Input: part model. Units: mm. Frame: model coordinates. A direction names the side the tool comes from. Coordinates: 2 decimals unless noted, no trailing zeros. Loops run counter-clockwise (first coordinate to the right, second up) from the corner with the lowest first, then second, coordinate; pieces in that order, holes last. Notation, with made-up numbers: (7, -17.75) - (32, -17.75) arc R6 cw to (32, -11.75) - close; hole circle Ø10 at (-27, -39.5). An arc over 180 degrees is marked (long way). Answer as CSV lines item,"result". Start each with the question number.
Autodesk Inventor part; units mm, degrees
ref_plane "YZ Plane" through (0, 0, 0) normal (1, 0, 0) x (0, 1, 0)
ref_plane "XZ Plane" through (0, 0, 0) normal (0, 1, 0) x (-1, 0, 0)
ref_plane "XY Plane" through (0, 0, 0) normal (0, 0, 1) x (1, 0, 0)
sketch "Sketch1" plane through (0, 0, 0) normal (0, 0, 1) x (1, 0, 0)
  circle A0 centre (0, 0) radius 40.5
  arc A1 (-25.4, 37.7504) -> (25.4, 37.7504) centre (0, 0) ccw
  line L0 (-25.4, 37.7504) -> (-25.4, 57.7504)
  line L1 (-25.4, 57.7504) -> (25.4, 57.7504)
  line L2 (25.4, 57.7504) -> (25.4, 37.7504)
  dimension "d1" = 5
  dimension "d9" = 20
extrude "Extrusion1" add sketch "Sketch1" along normal blind 12
sketch "Sketch2" plane through (-25.4, 57.7504, 0) normal (0, 1, 0) x (1, 0, 0)
  line L0 (0, -12) -> (50.8, -12)
  line L1 (50.8, -12) -> (50.8, 0)
  line L2 (50.8, 0) -> (0, 0)
  line L3 (0, 0) -> (0, -12)
  point P0 (25.4, 0)
extrude "Extrusion2" add sketch "Sketch2" along normal blind 12
sketch "Sketch3" plane through (0, 0, 12) normal (0, 0, 1) x (1, 0, 0)
  line L0 (-25.4, 37.7504) -> (-25.4, 69.7504)
  line L1 (25.4, 37.7504) -> (25.4, 69.7504)
  line L2 (-25.4, 69.7504) -> (25.4, 69.7504)
  line L3 (25.4, 69.7504) -> (25.4, 56.7504)
  line L4 (25.4, 56.7504) -> (-25.4, 56.7504)
  line L5 (-25.4, 56.7504) -> (-25.4, 69.7504)
  point P0 (0, 0)
  dimension "d12" = 13
extrude "Extrusion3" add sketch "Sketch3" along normal blind 17.2
sketch "Sketch4" plane through (0, 0, 29.2) normal (0, 0, 1) x (1, 0, 0)
  line L0 (25.4, 69.7504) -> (-25.4, 69.7504)
  line L1 (-25.4, 69.7504) -> (-25.4, 37.7504)
  circle A0 centre (0, 0) radius 8.5
  arc A1 (-25.4, 37.7504) -> (25.4, 37.7504) centre (0, 0) ccw
  arc A2 (-25.4, 37.7504) -> (25.4, 37.7504) centre (0, 0) ccw
  line L2 (25.4, 37.7504) -> (25.4, 69.7504)
  line L3 (25.4, 37.7504) -> (25.4, 69.7504)
  line L4 (25.4, 69.7504) -> (-25.4, 69.7504)
  dimension "d15" = 17
extrude "Extrusion4" add sketch "Sketch4" along normal blind 5
sketch "Sketch5" plane through (0, 0, 34.2) normal (0, 0, 1) x (1, 0, 0)
  arc A0 (-25.4, 37.7504) -> (25.4, 37.7504) centre (0, 0) ccw
  circle A1 centre (0, 0) radius 4.5
  line L0 (-25.4, 37.7504) -> (-25.4, 69.7504)
  line L1 (-25.4, 37.7504) -> (-25.4, 69.7504)
  line L2 (25.4, 69.7504) -> (-25.4, 69.7504)
  line L3 (-25.4, 69.7504) -> (25.4, 69.7504)
  line L4 (25.4, 69.7504) -> (25.4, 37.7504)
  dimension "d18" = 9
extrude "Extrusion5" add sketch "Sketch5" along normal blind 27
sketch "Sketch6" plane through (0, 0, 61.2) normal (0, 0, 1) x (1, 0, 0)
  line L0 (25.4, 69.7504) -> (-25.4, 69.7504)
  line L1 (-25.4, 56.7504) -> (-25.4, 37.7504)
  line L2 (-25.4, 69.7504) -> (-25.4, 37.7504)
  line L3 (-25.4, 69.7504) -> (25.4, 69.7504)
  arc A0 (-25.4, 37.7504) -> (25.4, 37.7504) centre (0, 0) ccw
  line L4 (25.4, 37.7504) -> (25.4, 69.7504)
  arc A1 (-25.4, 37.7504) -> (25.4, 37.7504) centre (0, 0) ccw
  circle A2 centre (0, 0) radius 8.5
  dimension "d21" = 17
extrude "Extrusion6" add sketch "Sketch6" along normal blind 5
sketch "Sketch7" plane through (-25.4, 69.7504, 0) normal (0, 1, 0) x (1, 0, 0)
  line L0 (50.8, 0) -> (0, 0)
  line L1 (0, -29.2) -> (0, -66.2)
  line L2 (50.8, 0) -> (0, 0)
  line L3 (0, 0) -> (0, -66.2)
  line L4 (0, -66.2) -> (50.8, -66.2)
  line L5 (50.8, -66.2) -> (50.8, 0)
  point P0 (25.4, 0)
extrude "Extrusion7" add sketch "Sketch7" along normal blind 25.4
sketch "Sketch8" plane through (-25.4, 95.1504, 0) normal (0, 1, 0) x (1, 0, 0)
  line L0 (0, -66.2) -> (50.8, -66.2)
  line L1 (0, -66.2) -> (50.8, -66.2)
  line L2 (50.8, -66.2) -> (25.4, -66.2)
  line L3 (33.9, -66.2) -> (16.9, -66.2)
  line L4 (50.8, -29.2) -> (50.8, -66.2)
  line L5 (50.8, 0) -> (50.8, -12)
  line L6 (50.8, -66.2) -> (50.8, 0)
  line L7 (50.8, 0) -> (50.8, -33.1)
  line L8 (12.7, -20.4) -> (38.1, -20.4)
  line L9 (38.1, -20.4) -> (38.1, -45.8)
  line L10 (38.1, -45.8) -> (12.7, -45.8)
  line L11 (12.7, -45.8) -> (12.7, -20.4)
  line L12 (43.1, -15.4) -> (7.7, -15.4)
  line L13 (7.7, -15.4) -> (7.7, -50.8)
  line L14 (7.7, -50.8) -> (43.1, -50.8)
  line L15 (43.1, -50.8) -> (43.1, -15.4)
  point P0 (25.4, 0)
  dimension "d30" = 5
extrude "Extrusion8" cut sketch "Sketch8" against normal blind 25.4 contours L8 L9 L10 L11
properties part number "Tilt_Portion"
Item 1: Contact query for flat-ended pins moving along their axis: P1, Ø2, axis at y = 59, z = 20, coming from the -X side; P2, Ø1.5, axis at x = 22, y = 76.5, coming from the -Z side; P3, Ø17, axis at y = 75.5, z = 33, coming from the +X side; P4, Ø5, axis at x = -30, z = 15.5, coming from the +Y side. Output: stop coordinate, or through.
Item 2: Draft query along Y for faces 1 (the flat face through (4, -4, 61.2)), 2 (the flat face through (0, 45, 0)), 3 (the flat face through (0, 95.15, 18)). Return one class per face: pulls with the +Y half, pulls with the -Y half, needs draft (parallel to the pull), parting line crosses it, or undercut.
Item 3: Material intervals for probe 1 along Y at (x, z) = (0, 32.95); probe 2 along Z at (x, y) = (-11.5, 73.5); probe 3 along Y at (x, z) = (0, 55.75), sorted ascending.
Item 4: Section query D-D, the plane z = 53. Output: boundary loops of the cut face in (x, y), and give its area (3 significant figures).
Item 5: Section query C-C, the plane y = 0. Output: boundary loops of the cut face in (x, z).
Item 6: Section query B-B, the plane x = 0. Output: boundary loops of the cut face in (y, z).
Item 7: Section query A-A, the plane y = 45. Output: boundary loops of the cut face in (x, z), and give its area (3 significant figures).
Item 8: Set-up query: faces 4 (the flat face through (0, 83, 45.8)), 5 (the cylindrical face through (4.57, -7.167, 31.665)), 6 (the flat face through (0, 56.75, 20)), 7 (the cylindrical face through (4.57, -7.167, 63.665)). Return all of +Z, -Z, +X, -X, +Y, -Y with unobstructed straight access to the full face (end or side cutting, diameter ignored); none if empty.
Response values:
1,P1,"stops at x = -25.4"
1,P2,"stops at z = 0"
1,P3,"stops at x = 25.4"
1,P4,"passes through"
2,face 1,"undercut"
2,face 2,"needs draft"
2,face 3,"pulls with the +Y half"
3,probe 1,"y = -45.5 to -8.5, 8.5 to 69.75"
3,probe 2,"z = 0 to 20.4, 45.8 to 66.2"
3,probe 3,"y = -45.5 to -4.5, 4.5 to 95.15"
4,outline,"(-25.4, 37.75) arc R45.5 ccw (long way) to (25.4, 37.75) - (25.4, 95.15) - (-25.4, 95.15) - close; hole circle Ø9 at (0, 0)"
4,area,"9,090 mm²"
5,outline,"(-45.5, 0) - (-40.5, 0) - (-40.5, 12) - (-45.5, 12) - close; (-45.5, 29.2) - (-8.5, 29.2) - (-8.5, 34.2) - (-4.5, 34.2) - (-4.5, 61.2) - (-8.5, 61.2) - (-8.5, 66.2) - (-45.5, 66.2) - close; (4.5, 34.2) - (8.5, 34.2) - (8.5, 29.2) - (45.5, 29.2) - (45.5, 66.2) - (8.5, 66.2) - (8.5, 61.2) - (4.5, 61.2) - close; (40.5, 0) - (45.5, 0) - (45.5, 12) - (40.5, 12) - close"
6,outline,"(-45.5, 0) - (-40.5, 0) - (-40.5, 12) - (-45.5, 12) - close; (-45.5, 29.2) - (-8.5, 29.2) - (-8.5, 34.2) - (-4.5, 34.2) - (-4.5, 61.2) - (-8.5, 61.2) - (-8.5, 66.2) - (-45.5, 66.2) - close; (4.5, 34.2) - (8.5, 34.2) - (8.5, 29.2) - (56.75, 29.2) - (56.75, 12) - (40.5, 12) - (40.5, 0) - (95.15, 0) - (95.15, 20.4) - (69.75, 20.4) - (69.75, 45.8) - (95.15, 45.8) - (95.15, 66.2) - (8.5, 66.2) - (8.5, 61.2) - (4.5, 61.2) - close"
7,outline,"(-25.4, 0) - (25.4, 0) - (25.4, 12) - (-25.4, 12) - close; (-25.4, 29.2) - (25.4, 29.2) - (25.4, 66.2) - (-25.4, 66.2) - close"
7,area,"2,490 mm²"
8,face 4,"+Y"
8,face 5,"-Z"
8,face 6,"+X, -X, -Y"
8,face 7,"+Z"
